Verification items for the finished model (mm, model axes). A direction names the side the tool comes from. Coordinates: 2 decimals unless noted, no trailing zeros. Loops run counter-clockwise (first coordinate to the right, second up) from the corner with the lowest first, then second, coordinate; pieces in that order, holes last. Notation, with made-up numbers: (48.25, 72) -> (63.25, 72) arc R28 ccw to (63.25, 93) -> close; hole circle Ø9 at (-29.75, 19). An arc over 180 degrees is marked (long way). Write item = value, one per line.
```python
from build123d import *

# Parameters (mm, degrees)
BOSS_EXTRUDE1_DEPTH = 8
CUT_EXTRUDE1_DEPTH  = 8
SKETCH8_R           = 2.4
CUT_EXTRUDE4_DEPTH  = 21.892582416
SKETCH9_R           = 3.1
CUT_EXTRUDE5_DEPTH  = 1
CUT_EXTRUDE6_DEPTH  = 21.892582416
CUT_EXTRUDE7_DEPTH  = 21.892582416


with BuildPart() as part:
    # Sketch1 → Boss-Extrude1 (new body)
    with BuildSketch(Plane(origin=(0, 0, 0), x_dir=(1, 0, 0), z_dir=(0, 1, 0))):
        Polygon((-15.5, -3.5), (15.5, -3.5), (15.5, 3.5), (15.5, 11.5), (8.5, 11.5), (8.5, 3.5), (-15.5, 3.5), align=None)
    extrude(amount=BOSS_EXTRUDE1_DEPTH)

    # Sketch3 → Cut-Extrude1 (cut)
    with BuildSketch(Plane(origin=(0, 8, 0), x_dir=(1, 0, 0), z_dir=(0, 1, 0))):
        with BuildLine():
            ThreePointArc((-15.5, 0), (-14.474873734, 2.474873734), (-12, 3.5))
            Line((-12, 3.5), (-15.5, 3.5))
            Line((-15.5, 3.5), (-15.5, 0))
        make_face()
        with BuildLine():
            ThreePointArc((-12, -3.5), (-14.474873734, -2.474873734), (-15.5, 0))
            Line((-15.5, 0), (-15.5, -3.5))
            Line((-15.5, -3.5), (-12, -3.5))
        make_face()
        with BuildLine():
            ThreePointArc((15.5, 0), (14.474873734, -2.474873734), (12, -3.5))
            Line((12, -3.5), (15.5, -3.5))
            Line((15.5, -3.5), (15.5, 0))
        make_face()
        with BuildLine():
            Line((15.5, 11.5), (12, 11.5))
            ThreePointArc((12, 11.5), (14.474873734, 10.474873734), (15.5, 8))
            Line((15.5, 8), (15.5, 11.5))
        make_face()
        with BuildLine():
            Line((8.5, 11.5), (8.5, 8))
            ThreePointArc((8.5, 8), (9.525126266, 10.474873734), (12, 11.5))
            Line((12, 11.5), (8.5, 11.5))
        make_face()
    extrude(amount=-CUT_EXTRUDE1_DEPTH, mode=Mode.SUBTRACT)

    # Sketch8 → Cut-Extrude4 (cut, through all)
    with BuildSketch(Plane(origin=(0, 8, 0), x_dir=(1, 0, 0), z_dir=(0, 1, 0))):
        with Locations(Location((12, 8, 0), (0, 0, 270))):
            Circle(SKETCH8_R)
        with Locations(Location((12, 0, 0), (0, 0, 270))):
            Circle(SKETCH8_R)
        with Locations(Location((4, 0, 0), (0, 0, 270))):
            Circle(SKETCH8_R)
        with Locations(Location((-4, 0, 0), (0, 0, 270))):
            Circle(SKETCH8_R)
    extrude(amount=-CUT_EXTRUDE4_DEPTH, mode=Mode.SUBTRACT)

    # Sketch9 → Cut-Extrude5 (cut)
    with BuildSketch(Plane(origin=(0, 8, 0), x_dir=(1, 0, 0), z_dir=(0, 1, 0))):
        with Locations(Location((12, 8, 0), (0, 0, 270))):
            Circle(SKETCH9_R)
        with Locations(Location((12, 0, 0), (0, 0, 270))):
            Circle(SKETCH9_R)
        with Locations(Location((4, 0, 0), (0, 0, 270))):
            Circle(SKETCH9_R)
        with Locations(Location((-4, 0, 0), (0, 0, 270))):
            Circle(SKETCH9_R)
    cut_extrude5 = extrude(amount=-CUT_EXTRUDE5_DEPTH, mode=Mode.SUBTRACT)

    # Mirror1: Cut-Extrude5 across plane
    add(cut_extrude5.mirror(Plane.ZX.offset(4)), mode=Mode.SUBTRACT)

    # Sketch10 → Cut-Extrude6 (cut, through all)
    with BuildSketch(Plane(origin=(0, 8, 0), x_dir=(1, 0, 0), z_dir=(0, 1, 0))):
        with BuildLine():
            ThreePointArc((9.389900826, 4.865957447), (9.25, 4), (9.389900826, 3.134042553))
            ThreePointArc((9.389900826, 3.134042553), (9.641748912, 2.880966401), (9.995419806, 2.929873418))
            ThreePointArc((9.995419806, 2.929873418), (12, 3.55), (14.004580194, 2.929873418))
            ThreePointArc((14.004580194, 2.929873418), (14.358251088, 2.880966401), (14.610099174, 3.134042553))
            ThreePointArc((14.610099174, 3.134042553), (14.75, 4), (14.610099174, 4.865957447))
            ThreePointArc((14.610099174, 4.865957447), (14.358251088, 5.119033599), (14.004580194, 5.070126582))
            ThreePointArc((14.004580194, 5.070126582), (12, 4.45), (9.995419806, 5.070126582))
            ThreePointArc((9.995419806, 5.070126582), (9.641748912, 5.119033599), (9.389900826, 4.865957447))
        make_face()
        with BuildLine():
            ThreePointArc((7.134042553, -2.610099174), (8, -2.75), (8.865957447, -2.610099174))
            ThreePointArc((8.865957447, -2.610099174), (9.119033599, -2.358251088), (9.070126582, -2.004580194))
            ThreePointArc((9.070126582, -2.004580194), (8.45, 0), (9.070126582, 2.004580194))
            ThreePointArc((9.070126582, 2.004580194), (9.119033599, 2.358251088), (8.865957447, 2.610099174))
            ThreePointArc((8.865957447, 2.610099174), (8, 2.75), (7.134042553, 2.610099174))
            ThreePointArc((7.134042553, 2.610099174), (6.880966401, 2.358251088), (6.929873418, 2.004580194))
            ThreePointArc((6.929873418, 2.004580194), (7.55, 0), (6.929873418, -2.004580194))
            ThreePointArc((6.929873418, -2.004580194), (6.880966401, -2.358251088), (7.134042553, -2.610099174))
        make_face()
        with BuildLine():
            ThreePointArc((-0.865957447, -2.610099174), (0, -2.75), (0.865957447, -2.610099174))
            ThreePointArc((0.865957447, -2.610099174), (1.119033599, -2.358251088), (1.070126582, -2.004580194))
            ThreePointArc((1.070126582, -2.004580194), (0.45, 0), (1.070126582, 2.004580194))
            ThreePointArc((1.070126582, 2.004580194), (1.119033599, 2.358251088), (0.865957447, 2.610099174))
            ThreePointArc((0.865957447, 2.610099174), (0, 2.75), (-0.865957447, 2.610099174))
            ThreePointArc((-0.865957447, 2.610099174), (-1.119033599, 2.358251088), (-1.070126582, 2.004580194))
            ThreePointArc((-1.070126582, 2.004580194), (-0.45, 0), (-1.070126582, -2.004580194))
            ThreePointArc((-1.070126582, -2.004580194), (-1.119033599, -2.358251088), (-0.865957447, -2.610099174))
        make_face()
        with BuildLine():
            ThreePointArc((-8.865957447, -2.610099174), (-8, -2.75), (-7.134042553, -2.610099174))
            ThreePointArc((-7.134042553, -2.610099174), (-6.880966401, -2.358251088), (-6.929873418, -2.004580194))
            ThreePointArc((-6.929873418, -2.004580194), (-7.55, 0), (-6.929873418, 2.004580194))
            ThreePointArc((-6.929873418, 2.004580194), (-6.880966401, 2.358251088), (-7.134042553, 2.610099174))
            ThreePointArc((-7.134042553, 2.610099174), (-8, 2.75), (-8.865957447, 2.610099174))
            ThreePointArc((-8.865957447, 2.610099174), (-9.119033599, 2.358251088), (-9.070126582, 2.004580194))
            ThreePointArc((-9.070126582, 2.004580194), (-8.45, 0), (-9.070126582, -2.004580194))
            ThreePointArc((-9.070126582, -2.004580194), (-9.119033599, -2.358251088), (-8.865957447, -2.610099174))
        make_face()
    extrude(amount=-CUT_EXTRUDE6_DEPTH, mode=Mode.SUBTRACT)

    # Sketch11 → Cut-Extrude7 (cut, through all)
    with BuildSketch(Plane(origin=(0, 8, 0), x_dir=(1, 0, 0), z_dir=(0, 1, 0))):
        with BuildLine():
            Line((-13.24, 0.84), (-14.177705214, 0.84))
            ThreePointArc((-14.177705214, 0.84), (-14.235940121, 0.821293884), (-14.27238805, 0.772173913))
            ThreePointArc((-14.27238805, 0.772173913), (-14.4, 0), (-14.27238805, -0.772173913))
            ThreePointArc((-14.27238805, -0.772173913), (-14.235940121, -0.821293884), (-14.177705214, -0.84))
            Line((-14.177705214, -0.84), (-13.24, -0.84))
            ThreePointArc((-13.24, -0.84), (-12.957157288, -0.957157288), (-12.84, -1.24))
            Line((-12.84, -1.24), (-12.84, -2.177705214))
            ThreePointArc((-12.84, -2.177705214), (-12.821293884, -2.235940121), (-12.772173913, -2.27238805))
            ThreePointArc((-12.772173913, -2.27238805), (-12, -2.4), (-11.227826087, -2.27238805))
            ThreePointArc((-11.227826087, -2.27238805), (-11.178706116, -2.235940121), (-11.16, -2.177705214))
            Line((-11.16, -2.177705214), (-11.16, -1.24))
            ThreePointArc((-11.16, -1.24), (-11.042842712, -0.957157288), (-10.76, -0.84))
            Line((-10.76, -0.84), (-9.822294786, -0.84))
            Line((-9.822294786, -0.84), (-9.751800721, -0.84))
            Line((-9.751800721, -0.84), (-8.55081169, -0.84))
            ThreePointArc((-8.55081169, -0.84), (-8.45, 0), (-8.55081169, 0.84))
            Line((-8.55081169, 0.84), (-9.751800721, 0.84))
            Line((-9.751800721, 0.84), (-9.822294786, 0.84))
            Line((-9.822294786, 0.84), (-10.76, 0.84))
            ThreePointArc((-10.76, 0.84), (-11.042842712, 0.957157288), (-11.16, 1.24))
            Line((-11.16, 1.24), (-11.16, 2.177705214))
            ThreePointArc((-11.16, 2.177705214), (-11.178706116, 2.235940121), (-11.227826087, 2.27238805))
            ThreePointArc((-11.227826087, 2.27238805), (-12, 2.4), (-12.772173913, 2.27238805))
            ThreePointArc((-12.772173913, 2.27238805), (-12.821293884, 2.235940121), (-12.84, 2.177705214))
            Line((-12.84, 2.177705214), (-12.84, 1.24))
            ThreePointArc((-12.84, 1.24), (-12.957157288, 0.957157288), (-13.24, 0.84))
        make_face()
    extrude(amount=-CUT_EXTRUDE7_DEPTH, mode=Mode.SUBTRACT)


solid = part.part
```
1) Release check for a two-part mould opening along X. For faces 5 (the face through (14.5, 4.06, 2.45)), 6 (the face through (-11.16, 4, -2)), 7 (the face through (0, 4, 3.5)) record: pulls with the +X half, pulls with the -X half, needs draft (parallel to the pull), parting line crosses it, or undercut.
Ans:
face_5 = pulls with the +X half
face_6 = undercut
face_7 = needs draft
2) Depth check by flat-ended pin: pin 1 Ø1 at (y, z) = (4.5, -2) entering from -X; pin 2 Ø5 at (x, z) = (12.5, -7.5) entering from -Y; pin 3 Ø2.5 at (x, y) = (1.5, 2.5) entering from -Z; pin 4 Ø1.9 at (x, z) = (13.5, -9) entering from +Y. Enter the tip coordinate at first touch or a pass-through.
Ans:
pin_1 = -15.16
pin_2 = 0
pin_3 = -3.5
pin_4 = 7
3) Sectioned sample at B-B, the plane x = 13.5. Count the separate pieces of the cut face and the enclosed holes in it, plus the area to 3 significant figures.
Ans:
separate_pieces = 4
enclosed_holes = 0
area = 35.4 mm2
4) Tool access check on faces 1 (the face through (0.45, 4.06, 0.03)), 2 (the face through (-2, 4, -3.5)), 3 (the face through (14.61, 0.49, 1.67)), 4 (the face through (7.074, 7.507, -0.404)). Record the directions out of +Z, -Z, +X, -X, +Y, -Y that give a thin tool (end or side, any length) a straight path to the whole face; none if there is none.
Ans:
face_1 = +Y, -Y
face_2 = -Z, -X, +Y, -Y
face_3 = -Y
face_4 = +Y
5) Sectioned sample at A-A, the plane x = -4. Record the cut outline in (y, z), plus the area to 3 significant figures.
Ans:
outline = (0, -3.5) -> (8, -3.5) -> (8, -3.1) -> (7, -3.1) -> (7, -2.4) -> (1, -2.4) -> (1, -3.1) -> (0, -3.1) -> close; (0, 3.1) -> (1, 3.1) -> (1, 2.4) -> (7, 2.4) -> (7, 3.1) -> (8, 3.1) -> (8, 3.5) -> (0, 3.5) -> close
area = 14.8 mm2
6) Material ranges on line 1 (Z direction, x = 8, y = 5.25); line 2 (X direction, y = 4.25, z = -4.75); line 3 (X direction, y = 0.4, z = -8), recorded low to high.
Ans:
line_1 = -3.5 to -2.75, 2.75 to 3.5
line_2 = 8.5 to 9.35, 10.57 to 13.43, 14.65 to 15.5
line_3 = 8.5 to 8.9, 15.1 to 15.5
